The listing builds one solid part. Answer for the finished solid, in the listing's coordinates (mm). A direction names the side the tool comes from. Give positions to 0.01 mm unless a question says otherwise; leave off trailing zeros. Write each loop counter-clockwise with the first axis right and the second up, starting at its lowest first coordinate (ties: lowest second). Pieces come first, ordered by that corner, then holes. Notation, with made-up numbers: M 35,-25 L 68,-25 A26 cw 68,10 Z; hole C 49.25,-9.75 d8. An arc over 180 degrees is marked long. Return JSON: item names as keys, results as strings.
from build123d import *

# Parameters (mm, degrees)
BASE_EXTRUSION_DEPTH    = 10.8
CONG_1_R                = 2
CONG_3_R                = 2
ENL_V_MAT_EXTRU_4_DEPTH = 9
ESQUISSE7_W             = 8.2
ESQUISSE7_H             = 10.06
ENL_V_MAT_EXTRU_5_DEPTH = 9
ESQUISSE8_R             = 2
ESQUISSE8_R_2           = 1.75
ENL_V_MAT_EXTRU_6_DEPTH = 56.825441717


with BuildPart() as part:
    # Esquisse1 → Base-Extrusion (new body)
    with BuildSketch(Plane.XY):
        with BuildLine():
            Line((0, 49), (0, 0))
            ThreePointArc((0, 0), (5, -5), (10, 0))
            Line((10, 0), (10, 49))
            ThreePointArc((10, 49), (5, 54), (0, 49))
        make_face()
    extrude(amount=BASE_EXTRUSION_DEPTH)

    # Congé1
    cong_1_edges = [part.edges().sort_by_distance(p)[0] for p in [
        (5, -5, 10.8),
        (10, 24.5, 10.8),
        (5, 54, 10.8),
        (0, 24.5, 10.8),
    ]]
    fillet(cong_1_edges, radius=CONG_1_R)

    # Congé3
    cong_3_edges = [part.edges().sort_by_distance(p)[0] for p in [
        (10, 24.5, 0),
        (5, -5, 0),
        (0, 24.5, 0),
        (5, 54, 0),
    ]]
    fillet(cong_3_edges, radius=CONG_3_R)

    # Esquisse6 → Enlèv. mat.-Extru.4 (cut)
    with BuildSketch(Plane(origin=(10, 0, 0), x_dir=(0, 0, -1), z_dir=(1, 0, 0))):
        Polygon((-9.5, 58.014149953), (-9.5, -9.353860788), (-1.3, -9.353860788), (-1.3, 56.548715687), align=None)
    extrude(amount=-ENL_V_MAT_EXTRU_4_DEPTH, mode=Mode.SUBTRACT)

    # Esquisse7 → Enlèv. mat.-Extru.5 (cut)
    with BuildSketch(Plane.ZY):
        with Locations((5.4, 0.429072807)):
            Rectangle(ESQUISSE7_W, ESQUISSE7_H)
    extrude(amount=-ENL_V_MAT_EXTRU_5_DEPTH, mode=Mode.SUBTRACT)

    # Esquisse8 → Enlèv. mat.-Extru.6 (cut, through all)
    with BuildSketch(Plane(origin=(0, 0, 0), x_dir=(-1, 0, 0), z_dir=(0, 0, -1))):
        with Locations((-5, 0)):
            Circle(ESQUISSE8_R)
        with Locations((-5, 49)):
            Circle(ESQUISSE8_R_2)
    extrude(amount=-ENL_V_MAT_EXTRU_6_DEPTH, mode=Mode.SUBTRACT)


solid = part.part
Item 1: A cutting plane is placed at B-B, the plane y = 45. Write down the section's boundary in (x, z).
Geometry results:
{"outline": "M 0,2 A2 ccw 2,0 L 8,0 A2 ccw 9.87,1.3 L 1,1.3 L 1,9.5 L 9.87,9.5 A2 ccw 8,10.8 L 2,10.8 A2 ccw 0,8.8 Z"}
Item 2: Which of the six approach directions +Z, -Z, +X, -X, +Y, -Y give full straight-line access (tool end or side, diameter ignored) to faces 4 (the cylindrical face through (5.38, 47.29, 10.14)), 5 (the flat face through (1, 29, 5))?
Geometry results:
{"face 4": "+Z, -Z", "face 5": "+X, +Y, -Y"}
Item 3: Find the intervals of material crossed by line 1 (Z direction, x = 6.25, y = 36.5); line 2 (Y direction, x = 5, z = 0.5); line 3 (Y direction, x = 5, z = 0.9), in increasing order.
Geometry results:
{"line 1": "z = 0 to 1.3, 9.5 to 10.8", "line 2": "y = -4.32 to -2, 2 to 47.25, 50.75 to 53.32", "line 3": "y = -4.67 to -2, 2 to 47.25, 50.75 to 53.67"}
Item 4: A cutting plane is placed at A-A, the plane x = 5. Write down the section's boundary in (y, z).
Geometry results:
{"outline": "M -4.87,1.3 A2 ccw -3,0 L -2,0 L -2,1.3 Z; M -4.87,9.5 L -2,9.5 L -2,10.8 L -3,10.8 A2 ccw Z; M 2,0 L 47.25,0 L 47.25,1.3 L 2,1.3 Z; M 2,9.5 L 47.25,9.5 L 47.25,10.8 L 2,10.8 Z; M 50.75,0 L 52,0 A2 ccw 53.87,1.3 L 50.75,1.3 Z; M 50.75,9.5 L 53.87,9.5 A2 ccw 52,10.8 L 50.75,10.8 Z"}
Item 5: Determine the mould class of faces 1 (the flat face through (0, 28, 5)), 2 (the cylindrical face through (6.6, -1.2, 10.1)), 3 (the flat face through (0.5, 5.459, 5.3)) for opening direction Y: +Y half, -Y half, draft (parallel to the pull), parting line (faces both ways), or undercut.
Geometry results:
{"face 1": "draft", "face 2": "undercut", "face 3": "-Y half"}
Item 6: Given pin 1 Ø1 at (y, z) = (8.5, 2.5) entering from +X; pin 2 Ø0.8 at (x, z) = (0.5, 6) entering from -Y, each flat-ended and moving along its own axis, determine where each tip first touches the part or whether it passes through.
Geometry results:
{"pin 1": "stops at x = 1", "pin 2": "stops at y = 5.46"}
